The model under review builds one solid part; all positions refer to its coordinate system, in mm. Face numbers are marked on the shaded views. A direction names the side the tool comes from. Coordinates: 2 decimals unless noted, no trailing zeros. Write each loop counter-clockwise with the first axis right and the second up, starting at its lowest first coordinate (ties: lowest second). Pieces come first, ordered by that corner, then holes. Notation, with made-up numbers: (8.5, 46.5) -> (62.5, 46.5) arc R17 cw to (62.5, 61.5) -> close; hole circle Ø7 at (59, 78). An arc over 180 degrees is marked (long way). Write each question's results on one line, items separated by ' | '.
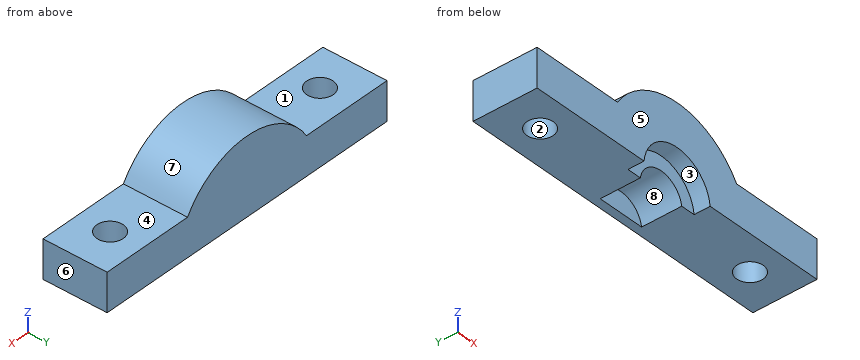
Autodesk Inventor part; units mm, degrees
ref_plane "YZ Plane" through (0, 0, 0) normal (1, 0, 0) x (0, 1, 0)
ref_plane "XZ Plane" through (0, 0, 0) normal (0, 1, 0) x (-1, 0, 0)
ref_plane "XY Plane" through (0, 0, 0) normal (0, 0, 1) x (1, 0, 0)
sketch "Schizzo1" plane through (0, 0, 0) normal (0, 1, 0) x (-1, 0, 0)
  line L0 (40, -9.5) -> (-40, -9.5)
  line L1 (-40, -9.5) -> (-40, 9.5)
  line L2 (-40, 9.5) -> (40, 9.5)
  line L3 (40, 9.5) -> (40, -9.5)
  line L4 (40, -9.5) -> (-40, 9.5) construction
  line L5 (-40, -9.5) -> (40, 9.5) construction
  point P0 (0, 0)
  point P1 (0, 0)
  point P2 (0, 0)
  dimension "d0" = 19
  dimension "d15" = 80
extrude "Estrusione1" add sketch "Schizzo1" along normal blind 16
sketch "Schizzo2" plane through (0, 0, 0) normal (0, -1, 0) x (1, 0, 0)
  line L0 (40, -9.5) -> (-40, -9.5)
  line L1 (0, -9.5) -> (0, -10.5)
  line L2 (0, -9.5) -> (1, -9.5) construction
  circle A0 centre (0, -10.5) radius 9.5
  point P0 (0, 0)
  dimension "d9" = 1
  dimension "d10" = 90
  dimension "d11" = 19
extrude "Estrusione2" cut sketch "Schizzo2" against normal blind 4
sketch "Schizzo3" plane through (0, 4, 0) normal (0, -1, 0) x (1, 0, 0)
  line L0 (9.4472, -9.5) -> (-9.4472, -9.5)
  line L1 (0, -9.5) -> (0, -10.5)
  line L2 (0, -9.5) -> (1, -9.5) construction
  circle A0 centre (0, -10.5) radius 6
  point P0 (0, 0)
  point P1 (9.5, -24.5)
  point P2 (-9.5, -24.5)
  point P3 (-9.4472, -9.5)
  dimension "d12" = 1
  dimension "d13" = 90
  dimension "d14" = 12
extrude "Estrusione3" cut sketch "Schizzo3" against normal blind 10
sketch "Schizzo5" plane through (0, 16, 0) normal (0, 1, 0) x (1, 0, 0)
  line L0 (40, 9.5) -> (-40, 9.5)
  line L1 (0, 9.5) -> (0, 10.5)
  line L2 (0, 9.5) -> (1, 9.5) construction
  circle A0 centre (0, 10.5) radius 20
  line L3 (40, -9.5) -> (40, 9.5)
  line L4 (-40, -9.5) -> (40, -9.5)
  line L5 (0, -9.5) -> (40, -9.5)
  line L6 (40, -9.5) -> (40, 9.5)
  line L7 (40, 0) -> (17.022, 0)
  line L8 (0, -9.5) -> (-40, -9.5)
  line L9 (-40, -9.5) -> (-40, -0.0448)
  line L10 (-40, 9.5) -> (-40, -9.5)
  line L11 (-40, -9.5) -> (-40, -0.0448)
  line L12 (-16.9943, -0.0448) -> (-40, -0.0448)
  point P0 (0, 0)
  dimension "d16" = 1
  dimension "d17" = 90
extrude "Estrusione4" cut sketch "Schizzo5" against normal blind 30 contours L3 L4 A0 L7 | L4 L9 L12 A0
sketch "Schizzo6" plane through (-40, 16, 0.0448) normal (0, 0, 1) x (1, 0, 0)
  line L0 (40, -16) -> (40, -8)
  line L1 (40, -16) -> (48, -16) construction
  line L2 (40, -8) -> (10, -8)
  line L3 (40, -8) -> (70, -8)
  line L4 (40, -8) -> (70, -8) construction
  dimension "d20" = 8
  dimension "d21" = 90
  dimension "d22" = 30
  dimension "d23" = 90
  dimension "d24" = 30
  dimension "d25" = 0
hole "Foro1" at (30, 8, 0.0448) at (-30, 8, 0.0448) direction (0, 0, -1) diameter 6.6 end through all
properties part number "14_base_avanti"
Q1. Add section D-D (x = -30). Write out the cut boundary in (y, z), plus the area to 3 significant figures.
Solution:
outline: (0, -9.5) -> (4.7, -9.5) -> (4.7, 0.04) -> (0, 0.04) -> close; (11.3, -9.5) -> (16, -9.5) -> (16, 0.04) -> (11.3, 0.04) -> close | area: 89.7 mm²
Q2. Add section A-A (x = 30). Write out the cut boundary in (y, z).
Solution:
outline: (0, -9.5) -> (4.7, -9.5) -> (4.7, 0) -> (0, 0) -> close; (11.3, -9.5) -> (16, -9.5) -> (16, 0) -> (11.3, 0) -> close
Q3. Clearance check with flat-ended pins moving along their axes: P1, Ø8, axis at x = 25.5, y = 6, coming from the +Z side; P2, Ø5.5, axis at x = 30, y = 8, coming from the -Z side; P3, Ø4, axis at x = 3, z = -8, coming from the -Y side; P4, Ø4.5, axis at x = 0, z = -4, coming from the -Y side. State where each tip first meets the part, or that it passes through.
Solution:
P1: z = 0 | P2: through | P3: y = 14 | P4: y = 4
Q4. Draft analysis for pull direction X (two halves, no side actions). For the marked faces 6, 7 and 8, state which applies: pulls with the +X half, pulls with the -X half, needs draft (parallel to the pull), parting line crosses it, or undercut.
Solution:
face 6: pulls with the +X half | face 7: parting line crosses it | face 8: undercut
Q5. Add section C-C (z = -5.5). Write out the cut boundary in (x, y), plus the area to 3 significant figures.
Solution:
outline: (-40, 0) -> (-8.08, 0) -> (-8.08, 4) -> (-3.32, 4) -> (-3.32, 14) -> (3.32, 14) -> (3.32, 4) -> (8.08, 4) -> (8.08, 0) -> (40, 0) -> (40, 16) -> (-40, 16) -> close; hole circle Ø6.6 at (-30, 8); hole circle Ø6.6 at (30, 8) | area: 1,080 mm²
Q6. Machinability: for the marked faces 1, 2, 3, 4 and 5, which of the approach directions +Z, -Z, +X, -X, +Y, -Y give a long, thin tool a straight path to every point of the face, cutting with its end or side? Answer none if there is none.
Solution:
face 1: +Z, -X, +Y, -Y | face 2: +Z, -Z | face 3: -Z, -Y | face 4: +Z, +X, +Y, -Y | face 5: +Z, -Z, +X, -X, -Y
Q7. Add section B-B (y = 8). Write out the cut boundary in (x, z).
Solution:
outline: (-40, -9.5) -> (-33.3, -9.5) -> (-33.3, 0.04) -> (-40, 0.04) -> close; (-26.7, -9.5) -> (-5.92, -9.5) arc R6 cw to (5.92, -9.5) -> (26.7, -9.5) -> (26.7, 0) -> (17.02, 0) arc R20 ccw to (-16.99, 0.04) -> (-26.7, 0.04) -> close; (33.3, -9.5) -> (40, -9.5) -> (40, 0) -> (33.3, 0) -> close
Q8. For line 1 (X direction, y = 8, z = -3); line 2 (Y direction, x = 30, z = -4.5); line 3 (X direction, y = 8, z = -6.25), list the stretches that pass through material, from the lowest coordinate up. Write a range as from..to.
Solution:
line 1: -40..-33.3, -26.7..26.7, 33.3..40 | line 2: 0..4.7, 11.3..16 | line 3: -40..-33.3, -26.7..-4.24, 4.24..26.7, 33.3..40
